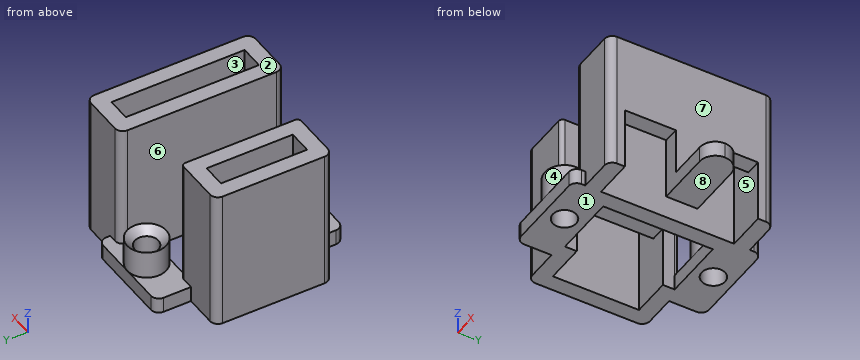
```python
from build123d import *

# Parameters (mm, degrees)
SKETCH001_W      = 8
SKETCH001_H      = 14
SKETCH001_W_2    = 3
SKETCH001_H_2    = 17
SKETCH001_H_3    = 11
PAD_DEPTH        = 2
SKETCH_R         = 2.5
PAD001_DEPTH     = 4
HOLE_D           = 3
HOLE_DEPTH       = 25
HOLE_CSINK_D     = 5.9
HOLE_CSINK_ANGLE = 90
SKETCH003_W      = 7
SKETCH003_H      = 15
SKETCH003_W_2    = 3
SKETCH003_H_2    = 11
SKETCH003_H_3    = 21
SKETCH003_H_4    = 17
PAD002_DEPTH     = 16
SKETCH004_W      = 6.5
SKETCH004_H      = 8
POCKET_DEPTH     = 2
SKETCH005_W      = 11
SKETCH005_H      = 8
POCKET001_DEPTH  = 2
FILLET_R         = 2
FILLET001_R      = 1.99
FILLET002_R      = 1
FILLET003_R      = 1
FILLET004_R      = 1
FILLET005_R      = 1
FILLET006_R      = 1
FILLET007_R      = 1
FILLET008_R      = 0.5
FILLET009_R      = 0.5
FILLET010_R      = 1
FILLET011_R      = 1
FILLET012_R      = 1
FILLET013_R      = 1


with BuildPart() as part:
    # Sketch001 → Pad (new body)
    with BuildSketch(Plane.XY):
        Polygon((6, 12), (-6, 12), (-6, 7.5), (-11, 7.5), (-11, -7.5), (-6, -7.5), (-6, -12), (6, -12), (6, -10.5), (11, -10.5), (11, -2), (18, -2), (18, 2), (11, 2), (11, 10.5), (6, 10.5), align=None)
        Rectangle(SKETCH001_W, SKETCH001_H, mode=Mode.SUBTRACT)
        with Locations((7.5, 0)):
            Rectangle(SKETCH001_W_2, SKETCH001_H_2, mode=Mode.SUBTRACT)
        with Locations((-7.5, 0)):
            Rectangle(SKETCH001_W_2, SKETCH001_H_3, mode=Mode.SUBTRACT)
    extrude(amount=PAD_DEPTH)

    # Sketch (on Face30 of Pad) → Pad001 (join)
    with BuildSketch(Plane.XY.offset(2)):
        with Locations((0, 9.5)):
            Circle(SKETCH_R)
        with Locations((0, -9.5)):
            Circle(SKETCH_R)
    extrude(amount=PAD001_DEPTH)

    # Hole
    with Locations(Plane.XY.offset(6)):
        with Locations((0, 9.5), (0, -9.5)):
            CounterSinkHole(HOLE_D / 2, HOLE_CSINK_D / 2, depth=HOLE_DEPTH, counter_sink_angle=HOLE_CSINK_ANGLE)

    # Sketch003 (on Face5 of Hole) → Pad002 (join)
    with BuildSketch(Plane.XY.offset(2)):
        with Locations((-7.5, 0)):
            Rectangle(SKETCH003_W, SKETCH003_H)
        with Locations((-7.5, 0)):
            Rectangle(SKETCH003_W_2, SKETCH003_H_2, mode=Mode.SUBTRACT)
        with Locations((7.5, 0)):
            Rectangle(SKETCH003_W, SKETCH003_H_3)
        with Locations((7.5, 0)):
            Rectangle(SKETCH003_W_2, SKETCH003_H_4, mode=Mode.SUBTRACT)
    extrude(amount=PAD002_DEPTH)

    # Sketch004 (on Face37 of Pad002) → Pocket (cut)
    with BuildSketch(Plane.YZ.offset(11)):
        with Locations((-5.25, 4)):
            Rectangle(SKETCH004_W, SKETCH004_H)
        with Locations((5.25, 4)):
            Rectangle(SKETCH004_W, SKETCH004_H)
    extrude(amount=-POCKET_DEPTH, mode=Mode.SUBTRACT)

    # Sketch005 (on Face37 of Pocket) → Pocket001 (cut)
    with BuildSketch(Plane.YZ.offset(-4)):
        with Locations((0, 4)):
            Rectangle(SKETCH005_W, SKETCH005_H)
    extrude(amount=-POCKET001_DEPTH, mode=Mode.SUBTRACT)

    # Fillet
    fillet_edges = [part.edges().sort_by_distance(p)[0] for p in [
        (18, 2, 1),
    ]]
    fillet(fillet_edges, radius=FILLET_R)

    # Fillet001
    fillet001_edges = [part.edges().sort_by_distance(p)[0] for p in [
        (18, -2, 1),
    ]]
    fillet(fillet001_edges, radius=FILLET001_R)

    # Fillet002
    fillet002_edges = [part.edges().sort_by_distance(p)[0] for p in [
        (11, 10.5, 10),
    ]]
    fillet(fillet002_edges, radius=FILLET002_R)

    # Fillet003
    fillet003_edges = [part.edges().sort_by_distance(p)[0] for p in [
        (11, -10.5, 10),
    ]]
    fillet(fillet003_edges, radius=FILLET003_R)

    # Fillet004
    fillet004_edges = [part.edges().sort_by_distance(p)[0] for p in [
        (4, -10.5, 10),
    ]]
    fillet(fillet004_edges, radius=FILLET004_R)

    # Fillet005
    fillet005_edges = [part.edges().sort_by_distance(p)[0] for p in [
        (4, 10.5, 10),
    ]]
    fillet(fillet005_edges, radius=FILLET005_R)

    # Fillet006
    fillet006_edges = [part.edges().sort_by_distance(p)[0] for p in [
        (-11, 7.5, 10),
    ]]
    fillet(fillet006_edges, radius=FILLET006_R)

    # Fillet007
    fillet007_edges = [part.edges().sort_by_distance(p)[0] for p in [
        (-11, -7.5, 10),
    ]]
    fillet(fillet007_edges, radius=FILLET007_R)

    # Fillet008
    fillet008_edges = [part.edges().sort_by_distance(p)[0] for p in [
        (-4, 7.5, 10),
    ]]
    fillet(fillet008_edges, radius=FILLET008_R)

    # Fillet009
    fillet009_edges = [part.edges().sort_by_distance(p)[0] for p in [
        (-4, -7.5, 10),
    ]]
    fillet(fillet009_edges, radius=FILLET009_R)

    # Fillet010
    fillet010_edges = [part.edges().sort_by_distance(p)[0] for p in [
        (-6, -12, 1),
    ]]
    fillet(fillet010_edges, radius=FILLET010_R)

    # Fillet011
    fillet011_edges = [part.edges().sort_by_distance(p)[0] for p in [
        (6, -12, 1),
    ]]
    fillet(fillet011_edges, radius=FILLET011_R)

    # Fillet012
    fillet012_edges = [part.edges().sort_by_distance(p)[0] for p in [
        (-6, 12, 1),
    ]]
    fillet(fillet012_edges, radius=FILLET012_R)

    # Fillet013
    fillet013_edges = [part.edges().sort_by_distance(p)[0] for p in [
        (6, 12, 1),
    ]]
    fillet(fillet013_edges, radius=FILLET013_R)


solid = part.part
```
Verification items for the finished model (mm, model axes). Face numbers are marked on the shaded views. A direction names the side the tool comes from. Round coordinates to 2 decimals unless told otherwise and drop trailing zeros. Write each loop counter-clockwise with the first axis right and the second up, starting at its lowest first coordinate (ties: lowest second). Pieces come first, ordered by that corner, then holes. Notation, with made-up numbers: (51, 74.5) -> (84, 74.5) arc R23 ccw to (84, 84.5) -> close; hole circle Ø11 at (-35, 19). An arc over 180 degrees is marked (long way). Write each question's results on one line, items separated by ' | '.
Q1. Sectioned sample at A-A, the plane x = -7.5. Record the boundary of the cut face in (y, z), and give its area (3 significant figures).
Derived:
outline: (-7.5, 0) -> (-5.5, 0) -> (-5.5, 18) -> (-7.5, 18) -> close; (5.5, 0) -> (7.5, 0) -> (7.5, 18) -> (5.5, 18) -> close | area: 72.0 mm²
Q2. Go/stop test with flat-tipped pins: pin 1 Ø8 at (x, y) = (1, -6) entering from -Z; pin 2 Ø1 at (x, y) = (10.5, 6.5) entering from -Z; pin 3 Ø5.5 at (x, z) = (12, 5) entering from -Y; pin 4 Ø1 at (y, z) = (-4.5, 7) entering from +X. Record where each tip stops, or that it passes through.
Derived:
pin 1: stops at z = 0 | pin 2: stops at z = 8 | pin 3: stops at y = -10.5 | pin 4: stops at x = 6
Q3. Draft check along X on the marked faces 6, 7 and 8. Enter one of: released by +X, released by -X, zero draft, split by the parting line, or undercut.
Derived:
face 6: undercut | face 7: released by +X | face 8: zero draft
Q4. Sectioned sample at C-C, the plane z = 13.75. Record the boundary of the cut face in (x, y).
Derived:
outline: (-11, -6.5) arc R1 ccw to (-10, -7.5) -> (-4.5, -7.5) arc R0.5 ccw to (-4, -7) -> (-4, 7) arc R0.5 ccw to (-4.5, 7.5) -> (-10, 7.5) arc R1 ccw to (-11, 6.5) -> close; (4, -9.5) arc R1 ccw to (5, -10.5) -> (10, -10.5) arc R1 ccw to (11, -9.5) -> (11, 9.5) arc R1 ccw to (10, 10.5) -> (5, 10.5) arc R1 ccw to (4, 9.5) -> close; hole (-9, -5.5) -> (-6, -5.5) -> (-6, 5.5) -> (-9, 5.5) -> close; hole (6, -8.5) -> (9, -8.5) -> (9, 8.5) -> (6, 8.5) -> close
Q5. Access from +Z, -Z, +X, -X, +Y, -Y to the whole of each face (thin tool, end or side, straight path). Record for the marked faces 1, 2, 3, 4 and 5.
Derived:
face 1: -Z, +X, -X, +Y, -Y | face 2: +Z, +X, -X, +Y, -Y | face 3: +Z, -Z | face 4: +Z | face 5: -Z
Q6. Sectioned sample at D-D, the plane x = 11.5. Record the boundary of the cut face in (y, z), and give its area (3 significant figures).
Derived:
outline: (-2, 0) -> (2, 0) -> (2, 2) -> (-2, 2) -> close | area: 8.00 mm²
Q7. Thickness scan on probe 1 along X at (y, z) = (-9.5, 2.2); probe 2 along X at (y, z) = (5.75, 12); probe 3 along X at (y, z) = (-3, 14.25). Record the ranges inside material, lowest first.
Derived:
probe 1: x = -2.5 to -1.5, 1.5 to 2.5, 4 to 11 | probe 2: x = -11 to -4, 4 to 6, 9 to 11 | probe 3: x = -11 to -9, -6 to -4, 4 to 6, 9 to 11
Q8. Sectioned sample at B-B, the plane y = -3. Record the boundary of the cut face in (x, z), and give its area (3 significant figures).
Derived:
outline: (-11, 0) -> (-9, 0) -> (-9, 18) -> (-11, 18) -> close; (-6, 8) -> (-4, 8) -> (-4, 18) -> (-6, 18) -> close; (4, 0) -> (6, 0) -> (6, 18) -> (4, 18) -> close; (9, 8) -> (11, 8) -> (11, 18) -> (9, 18) -> close | area: 112 mm²
